Input: part model. Units: mm. Frame: model coordinates. A direction names the side the tool comes from. Coordinates: 2 decimals unless noted, no trailing zeros. Write each loop counter-clockwise with the first axis right and the second up, starting at its lowest first coordinate (ties: lowest second). Pieces come first, ordered by that corner, then holes. Notation, with made-up numbers: M 39,5.5 L 88,5.5 A24 ccw 88,19.5 Z; hole C 11.5,32.25 d3. An arc over 180 degrees is marked long. Use CSV: the item, a comma, the result in double quotes.
```python
from build123d import *

# Parameters (mm, degrees)
EXTRUDE_1_DEPTH     = 4
SKETCH_2_W          = 12
SKETCH_2_H          = 5
EXTRUDE_2_DEPTH     = 20
SKETCH_6_R          = 4
CUT_EXTRUDE_5_DEPTH = 21


with BuildPart() as part:
    # 草图1 → 凸台-拉伸1 (new body)
    with BuildSketch(Plane.XY):
        Polygon((0.147281285, 10), (0.147281285, 70), (10.147281285, 80), (20.147281285, 70), (20.147281285, 10), (10.147281285, 0), align=None)
    extrude(amount=EXTRUDE_1_DEPTH)

    # 草图2 → 凸台-拉伸2 (add)
    with BuildSketch(Plane(origin=(0, 0, 0), x_dir=(-1, 0, 0), z_dir=(0, 0, -1))):
        with Locations((-10.147281285, 49.5)):
            Rectangle(SKETCH_2_W, SKETCH_2_H)
    extrude(amount=EXTRUDE_2_DEPTH)

    # 草图6 → 切除-拉伸5 (cut)
    with BuildSketch(Plane.XZ.offset(-47)):
        with Locations(Location((10.147281285, -13, 0), (0, 0, 270))):
            Circle(SKETCH_6_R)
        with BuildLine():
            Line((16.147281285, -20), (16.147281285, -13))
            ThreePointArc((16.147281285, -13), (10.147281285, -19), (4.147281285, -13))
            Line((4.147281285, -13), (4.147281285, -20))
            Line((4.147281285, -20), (16.147281285, -20))
        make_face()
    extrude(amount=-CUT_EXTRUDE_5_DEPTH, mode=Mode.SUBTRACT)


solid = part.part
```
1. Access query for faces 1 (the flat face through (10, 52, -7)), 2 (the flat face through (4.147, 49, -6)), 3 (the flat face through (16.147, 49, -6)). Directions: +Z, -Z, +X, -X, +Y, -Y. A direction counts if a zero-diameter tool reaches every point of the face in a straight line with its end or side. Return the directions, or none.
Resolved:
face 1,"-Z, +X, -X, +Y"
face 2,"-Z, -X, +Y, -Y"
face 3,"-Z, +X, +Y, -Y"
2. Section B-B (y = 46). Return loops of the section in (x, z), then the cut area to 3 significant figures.
Resolved:
outline,"M 0.15,0 L 20.15,0 L 20.15,4 L 0.15,4 Z"
area,"80.0 mm^2"
3. Section D-D (x = 2.75). Return loops of the section in (y, z), then the cut area to 3 significant figures.
Resolved:
outline,"M 7.4,0 L 72.6,0 L 72.6,4 L 7.4,4 Z"
area,"261 mm^2"
4. Section C-C (z = 1.75). Return loops of the section in (x, y), then the cut area to 3 significant figures.
Resolved:
outline,"M 0.15,10 L 10.15,0 L 20.15,10 L 20.15,70 L 10.15,80 L 0.15,70 Z"
area,"1,400 mm^2"
5. Section A-A (z = -12.25). Return loops of the section in (x, y), then the cut area to 3 significant figures.
Resolved:
outline,"M 4.15,47 L 6.22,47 L 6.22,52 L 4.15,52 Z; M 14.08,47 L 16.15,47 L 16.15,52 L 14.08,52 Z"
area,"20.7 mm^2"
6. Material intervals for line 1 (X direction, y = 49.85, z = -13); line 2 (Z direction, x = 5, y = 74); line 3 (Y direction, x = 6.5, z = -1), sorted ascending. Write a range as [from, to].
Resolved:
line 1,"x = [4.15, 6.15], [14.15, 16.15]"
line 2,"z = [0, 4]"
line 3,"y = [47, 52]"
7. Contact query for flat-ended pins moving along their axis: pin 1 Ø10.5 at (x, z) = (10.15, -13) entering from -Y; pin 2 Ø1.5 at (y, z) = (51.5, -8) entering from +X; pin 3 Ø8 at (x, z) = (4.5, -6.5) entering from +Y. Output: stop coordinate, or through.
Resolved:
pin 1,"stops at y = 47"
pin 2,"stops at x = 16.15"
pin 3,"stops at y = 52"
